For this review, take the finished solid that the model builds, in its own axes (mm). A direction names the side the tool comes from. Round coordinates to 2 decimals unless told otherwise and drop trailing zeros. Write each loop counter-clockwise with the first axis right and the second up, starting at its lowest first coordinate (ties: lowest second). Pieces come first, ordered by that corner, then holes. Notation, with made-up numbers: (53.25, 30.5) - (86.25, 30.5) arc R13 ccw to (86.25, 49.5) - close; hole circle Ø10 at (-33, -21). An arc over 180 degrees is marked (long way). One line per item, written item: value. Start each with the question number.
Q1. Tool access review of faces 4 (the face through (132, -6, 45)), 5 (the face through (132, -6, -45)), 6 (the face through (191, 62.653, 1)): name each direction out of +Z, -Z, +X, -X, +Y, -Y from which nothing blocks a thin tool from reaching the whole face with its end or side.
Q2. Add section A-A on x = 0. Write out the cut boundary in (y, z).
Q3. Add section B-B on z = 0. Write out the cut boundary in (x, y).
Q4. For probe 1 along Y at (x, z) = (0, -23); probe 2 along Y at (x, z) = (166, -31); probe 3 along Z at (x, y) = (78, -1.5) (3 decimals), list the stretches that pass through material, from the lowest coordinate up.
Q5. Mouldability with a two-part tool opening along Y and no side actions: class faces 1 (the face through (245.904, -71, 1)), 2 (the face through (41.39, -50.12, 0.7)), 3 (the face through (134.55, 1, 1)) as +Y half, -Y half, draft (parallel to the pull), parting line (faces both ways), or undercut.
Q6. Add section C-C on y = 9.5. Write out the cut boundary in (x, z), and give its area (3 significant figures).
Q7. Clearance check with flat-ended pins moving along their axes: pin 1 Ø10 at (x, z) = (-31, 23) entering from -Y; pin 2 Ø3 at (x, z) = (91.5, -20) entering from +Y; pin 3 Ø4 at (x, z) = (75.5, -20) entering from -Y. State where each tip first meets the part, or that it passes through.
Q8. Add section D-D on x = 171.5. Write out the cut boundary in (y, z).
```python
from build123d import *

# Parameters (mm, degrees)
SKETCH1_R                = 50
BOSS_EXTRUDE1_DEPTH      = 50
BOSS_EXTRUDE2_REACH      = 202
SKETCH2_R                = 45
BOSS_EXTRUDE3_DEPTH      = 45
BOSS_EXTRUDE3_DEPTH_BACK = 45


with BuildPart() as part:
    # Sketch1 → Boss-Extrude1 (new body, symmetric)
    with BuildSketch(Plane.XY):
        with BuildLine():
            Line((-80, 40), (-80, -40))
            Line((-80, -40), (-22.281665693, -61.061668614))
            ThreePointArc((-22.281665693, -61.061668614), (65, 0), (-22.281665693, 61.061668614))
            Line((-22.281665693, 61.061668614), (-80, 40))
        make_face()
        Circle(SKETCH1_R, mode=Mode.SUBTRACT)
    extrude(amount=BOSS_EXTRUDE1_DEPTH, both=True)

    # Sketch2 → Boss-Extrude2 (add, up to next)
    with BuildSketch(Plane(origin=(120, 0, 0), x_dir=(0, 0, -1), z_dir=(1, 0, 0)), mode=Mode.PRIVATE) as boss_extrude2_sk1:
        Circle(SKETCH2_R)
    boss_extrude2_tool1 = extrude(boss_extrude2_sk1.sketch, amount=-BOSS_EXTRUDE2_REACH, mode=Mode.PRIVATE) - part.part
    add(boss_extrude2_tool1.solids().sort_by_distance((120, 0, 0))[0])

    # Sketch3 → Boss-Extrude3 (add, two sides)
    with BuildSketch(Plane.XY) as boss_extrude3_sk:
        Polygon((120, 45), (120, 80.306694099), (245.903834127, 80.306694099), (245.903834127, 62.653347049), (134.550333897, 62.653347049), (134.550333897, -62.653347049), (245.903834127, -62.653347049), (245.903834127, -80.306694099), (120, -80.306694099), (120, -45), align=None)
    extrude(amount=BOSS_EXTRUDE3_DEPTH)
    extrude(boss_extrude3_sk.sketch, amount=-BOSS_EXTRUDE3_DEPTH_BACK)


solid = part.part
```
Result set:
1. face 4: +Z, +X, +Y, -Y
1. face 5: -Z, +X, +Y, -Y
1. face 6: +Z, -Z, +X
2. outline: (-65, -50) - (-50, -50) - (-50, 50) - (-65, 50) - close; (50, -50) - (65, -50) - (65, 50) - (50, 50) - close
3. outline: (-80, -40) - (-22.28, -61.06) arc R65 ccw to (46.9, -45) - (120, -45) - (120, -80.31) - (245.9, -80.31) - (245.9, -62.65) - (134.55, -62.65) - (134.55, 62.65) - (245.9, 62.65) - (245.9, 80.31) - (120, 80.31) - (120, 45) - (46.9, 45) arc R65 ccw to (-22.28, 61.06) - (-80, 40) - close; hole circle Ø100 at (0, 0)
4. probe 1: y = -65 to -50, 50 to 65
4. probe 2: y = -80.31 to -62.65, 62.65 to 80.31
4. probe 3: z = -44.975 to 44.975
5. face 1: draft
5. face 2: parting line
5. face 3: undercut
6. outline: (-80, -50) - (-49.09, -50) - (-49.09, 50) - (-80, 50) - close; (49.09, -50) - (64.3, -50) - (64.3, -43.99) - (120, -43.99) - (120, -45) - (134.55, -45) - (134.55, 45) - (120, 45) - (120, 43.99) - (64.3, 43.99) - (64.3, 50) - (49.09, 50) - close
6. area: 10,800 mm^2
7. pin 1: stops at y = -59.7
7. pin 2: stops at y = 41.02
7. pin 3: stops at y = -41.24
8. outline: (-80.31, -45) - (-62.65, -45) - (-62.65, 45) - (-80.31, 45) - close; (62.65, -45) - (80.31, -45) - (80.31, 45) - (62.65, 45) - close
